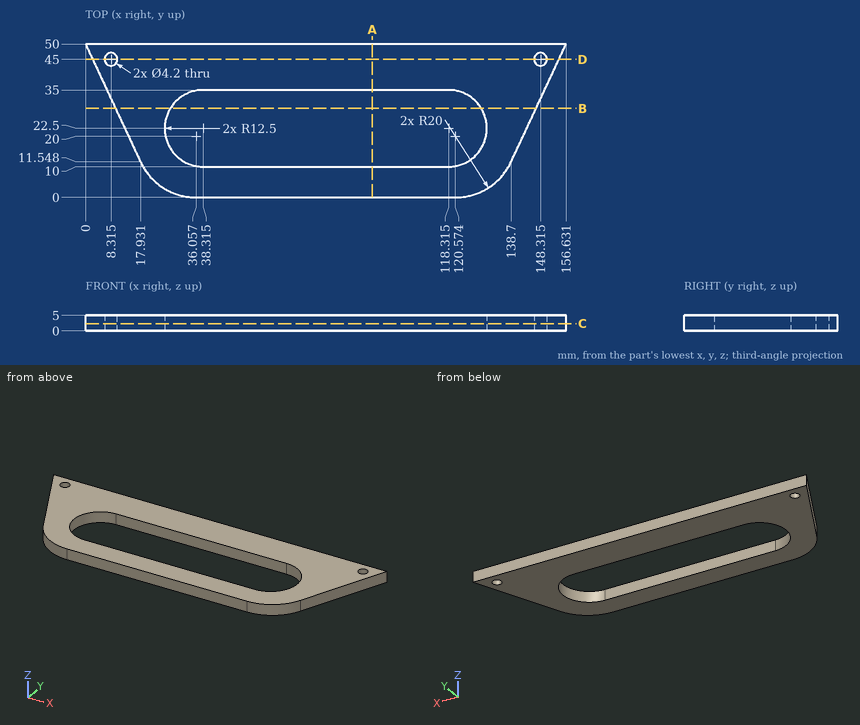
Geometry check sheet. Reference: drawing and pictorial views, mm from the part's lowest x, y, z. Give positions to 0.01 mm unless a question says otherwise; leave off trailing zeros. Order: outer loops, then holes, each group sorted by start corner. A loop starts at its lowest first (then second) coordinate and runs counter-clockwise, first axis right, second up. Notation, with made-up numbers: (2, 10.25) - (18, 10.25) arc R21 cw to (18, 21.25) - close; hole circle Ø7 at (47.25, -13). An arc over 180 degrees is marked (long way). Answer as CSV lines item,"result". Start each with the question number.
Item 1: Section check A-A, the plane x = 93.5. Record the boundary of the cut face in (y, z), plus the area to 3 significant figures.
Item 2: Section check C-C, the plane z = 2.35. Record the boundary of the cut face in (x, y) (1 decimal).
Item 3: Section check B-B, the plane y = 29. Record the boundary of the cut face in (x, z).
Item 4: Material ranges on L1, parallel to Y at x = 74.5, z = 2.65; L2, parallel to Y at x = 149.5, z = 1.35 (1 decimal); L3, parallel to X at y = 17, z = 1.45, recorded low to high.
Item 5: Section check D-D, the plane y = 45. Record the boundary of the cut face in (x, z) (1 decimal).
Filled in:
1,outline,"(0, 0) - (10, 0) - (10, 5) - (0, 5) - close; (35, 0) - (50, 0) - (50, 5) - (35, 5) - close"
1,area,"125 mm^2"
2,outline,"(0, 50) - (17.9, 11.5) arc R20 ccw to (36.1, 0) - (120.6, 0) arc R20 ccw to (138.7, 11.5) - (156.6, 50) - close; hole circle Ø4.2 at (8.3, 45); hole (38.3, 10) - (118.3, 10) arc R12.5 ccw to (118.3, 35) - (38.3, 35) arc R12.5 ccw to start; hole circle Ø4.2 at (148.3, 45)"
3,outline,"(9.79, 0) - (27.64, 0) - (27.64, 5) - (9.79, 5) - close; (128.99, 0) - (146.84, 0) - (146.84, 5) - (128.99, 5) - close"
4,L1,"0 to 10, 35 to 50"
4,L2,"34.7 to 43.3, 46.7 to 50"
4,L3,"15.39 to 27.09, 129.54 to 141.24"
5,outline,"(2.3, 0) - (6.2, 0) - (6.2, 5) - (2.3, 5) - close; (10.4, 0) - (146.2, 0) - (146.2, 5) - (10.4, 5) - close; (150.4, 0) - (154.3, 0) - (154.3, 5) - (150.4, 5) - close"
